Model file for the job. Use its own axes, mm. Round coordinates to 2 decimals unless told otherwise and drop trailing zeros. Order: outer loops, then holes, each group sorted by start corner. A loop starts at its lowest first (then second) coordinate and runs counter-clockwise, first axis right, second up. Notation, with made-up numbers: (57.25, 77) - (88.25, 77) arc R9 ccw to (88.25, 85) - close; hole circle Ø2 at (-34, -26.75). An arc over 180 degrees is marked (long way). Answer as CSV lines item,"result". Start each with the question number.
1. Band-saw the part on D-D on y = 57.15. List the corners of the cut face in (x, z) (3 decimals), then the cut area to 3 significant figures.
2. Pull direction X, two halves, no side cores. Call faces 1 (the face through (-19, 76.2, 0)), 2 (the face through (-38.1, 1, 0)), 3 (the face through (-19.59, -14.92, 0.04)), 4 (the face through (38.1, -39, 0)): released by +X, released by -X, zero draft, split by the parting line, or undercut.
3. Band-saw the part on C-C on x = 5.5. List the corners of the cut face in (y, z) (3 decimals).
4. Band-saw the part on A-A on y = -57.15. List the corners of the cut face in (x, z) (3 decimals), then the cut area to 3 significant figures.
5. Wall check: line 1 along Y through (x, z) = (-19.05, -2); line 2 along Y through (x, z) = (19.05, -1); line 3 along Y through (x, z) = (-20.5, 2.5). Give the ranges that are in metal, low to high. Write a range as [from, to].
6. Band-saw the part on B-B on z = -2. List the corners of the cut face in (x, y), then the cut area to 3 significant figures.
```python
from build123d import *

# Parameters (mm, degrees)
BOSS_EXTRUDE1_DEPTH      = 3.175
BOSS_EXTRUDE1_DEPTH_BACK = 3.175
SKETCH4_R                = 4.1656
CUT_EXTRUDE1_DEPTH       = 86.430512699


with BuildPart() as part:
    # Sketch3 → Boss-Extrude1 (new, two sides: drawn at the far end of the back side and taken through both)
    with BuildSketch(Plane.XY.offset(-BOSS_EXTRUDE1_DEPTH_BACK)):
        Polygon((0, 76.2), (-38.1, 76.2), (-38.1, -76.2), (38.1, -76.2), (38.1, 0), align=None)
    extrude(amount=BOSS_EXTRUDE1_DEPTH + BOSS_EXTRUDE1_DEPTH_BACK)

    # Sketch4 → Cut-Extrude1 (cut, through all)
    with BuildSketch(Plane.XY.offset(3.175)):
        with Locations((-19.05, -57.15)):
            Circle(SKETCH4_R)
        with Locations((19.05, -57.15)):
            Circle(SKETCH4_R)
        with Locations((19.05, -19.05)):
            Circle(SKETCH4_R)
        with Locations((-19.05, -19.05)):
            Circle(SKETCH4_R)
        with Locations((-19.05, 19.05)):
            Circle(SKETCH4_R)
        with Locations((-19.05, 57.15)):
            Circle(SKETCH4_R)
    extrude(amount=-CUT_EXTRUDE1_DEPTH, mode=Mode.SUBTRACT)


solid = part.part
```
Reply:
1,outline,"(-38.1, -3.175) - (-23.216, -3.175) - (-23.216, 3.175) - (-38.1, 3.175) - close; (-14.884, -3.175) - (9.525, -3.175) - (9.525, 3.175) - (-14.884, 3.175) - close"
1,area,"250 mm2"
2,face 1,"zero draft"
2,face 2,"released by -X"
2,face 3,"undercut"
2,face 4,"released by +X"
3,outline,"(-76.2, -3.175) - (65.2, -3.175) - (65.2, 3.175) - (-76.2, 3.175) - close"
4,outline,"(-38.1, -3.175) - (-23.216, -3.175) - (-23.216, 3.175) - (-38.1, 3.175) - close; (-14.884, -3.175) - (14.884, -3.175) - (14.884, 3.175) - (-14.884, 3.175) - close; (23.216, -3.175) - (38.1, -3.175) - (38.1, 3.175) - (23.216, 3.175) - close"
4,area,"378 mm2"
5,line 1,"y = [-76.2, -61.32], [-52.98, -23.22], [-14.88, 14.88], [23.22, 52.98], [61.32, 76.2]"
5,line 2,"y = [-76.2, -61.32], [-52.98, -23.22], [-14.88, 38.1]"
5,line 3,"y = [-76.2, -61.06], [-53.24, -22.96], [-15.14, 15.14], [22.96, 53.24], [61.06, 76.2]"
6,outline,"(-38.1, -76.2) - (38.1, -76.2) - (38.1, 0) - (0, 76.2) - (-38.1, 76.2) - close; hole circle Ø8.33 at (-19.05, -57.15); hole circle Ø8.33 at (-19.05, -19.05); hole circle Ø8.33 at (-19.05, 19.05); hole circle Ø8.33 at (-19.05, 57.15); hole circle Ø8.33 at (19.05, -57.15); hole circle Ø8.33 at (19.05, -19.05)"
6,area,"9,830 mm2"
